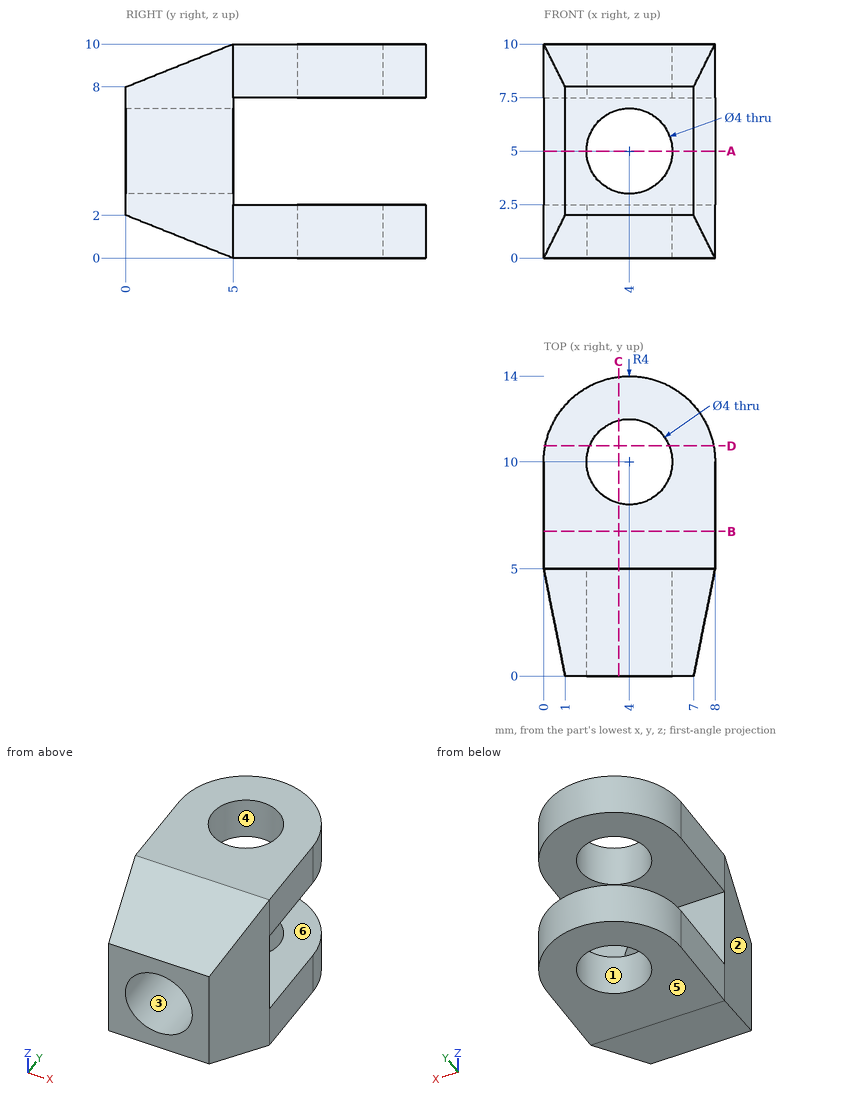
Design review of the part shown in the three views and the two pictorial views. Dimensions are in mm from the part's minimum x, y and z. A direction names the side the tool comes from. Coordinates: 2 decimals unless noted, no trailing zeros. Loops run counter-clockwise (first coordinate to the right, second up) from the corner with the lowest first, then second, coordinate; pieces in that order, holes last.
(1) Tool access review of the marked faces 5 and 6: name each direction out of +Z, -Z, +X, -X, +Y, -Y from which nothing blocks a thin tool from reaching the whole face with its end or side.
Determined:
face 5: -Z, +X, -X, +Y, -Y
face 6: +X, -X, +Y
(2) Insertion check: P1, Ø3.5, axis at x = 4, y = 10, coming from the -Z side; P2, Ø3, axis at x = 4, y = 2, coming from the +Z side; P3, Ø1.5, axis at x = 2.5, z = 5, coming from the +Y side. Each pin has a flat end and moves straight along its axis. Give the tip position at first contact, or say it passes through.
Determined:
P1: passes through
P2: stops at z = 9.4
P3: stops at y = 5
(3) Consider section D-D, the plane y = 10.75. Give the boundary of the cut face in (x, z).
Determined:
outline: (0.07, 0) - (2.15, 0) - (2.15, 2.5) - (0.07, 2.5) - close; (0.07, 7.5) - (2.15, 7.5) - (2.15, 10) - (0.07, 10) - close; (5.85, 0) - (7.93, 0) - (7.93, 2.5) - (5.85, 2.5) - close; (5.85, 7.5) - (7.93, 7.5) - (7.93, 10) - (5.85, 10) - close
(4) Consider section A-A, the plane z = 5. Give the boundary of the cut face in (x, y).
Determined:
outline: (0, 5) - (1, 0) - (2, 0) - (2, 5) - close; (6, 0) - (7, 0) - (8, 5) - (6, 5) - close
(5) Consider section B-B, the plane y = 6.75. Give the boundary of the cut face in (x, z), plus the area to 3 significant figures.
Determined:
outline: (0, 0) - (8, 0) - (8, 2.5) - (0, 2.5) - close; (0, 7.5) - (8, 7.5) - (8, 10) - (0, 10) - close
area: 40.0 mm2
(6) Draft analysis for pull direction Y (two halves, no side actions). For the marked faces 1, 2, 3 and 4, state which applies: +Y half, -Y half, draft (parallel to the pull), parting line (faces both ways), or undercut.
Determined:
face 1: undercut
face 2: -Y half
face 3: draft
face 4: undercut
(7) Wall thickness on L1, parallel to Z at x = 6.75, y = 12.5; L2, parallel to X at y = 10, z = 1.4; L3, parallel to Z at x = 4, y = 1.4: over which ranges is each line inside the solid? List them lowest first.
Determined:
L1: z = 0 to 2.5, 7.5 to 10
L2: x = 0 to 2, 6 to 8
L3: z = 1.44 to 3, 7 to 8.56
(8) Consider section C-C, the plane x = 3.5. Give the boundary of the cut face in (y, z), plus the area to 3 significant figures.
Determined:
outline: (0, 2) - (5, 0) - (8.06, 0) - (8.06, 2.5) - (5, 2.5) - (5, 3.06) - (0, 3.06) - close; (0, 6.94) - (5, 6.94) - (5, 7.5) - (8.06, 7.5) - (8.06, 10) - (5, 10) - (0, 8) - close; (11.94, 0) - (13.97, 0) - (13.97, 2.5) - (11.94, 2.5) - close; (11.94, 7.5) - (13.97, 7.5) - (13.97, 10) - (11.94, 10) - close
area: 46.1 mm2
